Input: part model. Units: mm. Frame: model coordinates. A direction names the side the tool comes from. Coordinates: 2 decimals unless noted, no trailing zeros. Order: outer loops, then holes, each group sorted by start corner. A loop starts at its lowest first (then second) coordinate and runs counter-clockwise, first axis right, second up.
from build123d import *

# Parameters (mm, degrees)
F1_DEPTH = 63.5
F2_DEPTH = 7.62
F4_DEPTH = 7.62
F5_R     = 7.735602
F6_DEPTH = 73.152
F5_R_2   = 7.041534
F7_DEPTH = 76.2


with BuildPart() as f1:
    # F0 (on Front) → F1 (new body)
    with BuildSketch(Plane.XZ):
        with BuildLine():
            Line((-11.978863, 32.654684), (-30.244743, 32.654684))
            Line((-30.244743, 32.654684), (-30.244743, -26.147846))
            Line((-30.244743, -26.147846), (51.452216, -26.147846))
            Line((51.452216, -26.147846), (51.452216, 32.654684))
            Line((51.452216, 32.654684), (33.186335, 32.654684))
            ThreePointArc((33.186335, 32.654684), (10.603736, 10.072085), (-11.978863, 32.654684))
        make_face()
        with BuildLine():
            Line((-4.722234, 32.654684), (-11.978863, 32.654684))
            ThreePointArc((-11.978863, 32.654684), (10.603736, 10.072085), (33.186335, 32.654684))
            Line((33.186335, 32.654684), (25.929707, 32.654684))
            ThreePointArc((25.929707, 32.654684), (10.603736, 17.328714), (-4.722234, 32.654684))
        make_face()
    extrude(amount=F1_DEPTH)

    # F0 (on Front) → F2 (join)
    with BuildSketch(Plane.XZ):
        with BuildLine():
            Line((-4.722234, 32.654684), (-11.978863, 32.654684))
            ThreePointArc((-11.978863, 32.654684), (10.603736, 10.072085), (33.186335, 32.654684))
            Line((33.186335, 32.654684), (25.929707, 32.654684))
            ThreePointArc((25.929707, 32.654684), (10.603736, 17.328714), (-4.722234, 32.654684))
        make_face()
    extrude(amount=-F2_DEPTH)

    # F3 (on face) → F4 (join)
    with BuildSketch(Plane.XZ.offset(63.5)):
        with BuildLine():
            ThreePointArc((-11.5002, 32.654684), (10.603736, 10.550748), (32.707673, 32.654684))
            Line((32.707673, 32.654684), (25.929707, 32.654684))
            ThreePointArc((25.929707, 32.654684), (10.603736, 17.328714), (-4.722234, 32.654684))
            Line((-4.722234, 32.654684), (-11.5002, 32.654684))
        make_face()
    extrude(amount=F4_DEPTH)

    # F5 (on face) → F6 (cut)
    with BuildSketch(Plane.XY.offset(32.654684)):
        with Locations((39.744381, -30.362099)):
            Circle(F5_R)
    extrude(amount=-F6_DEPTH, mode=Mode.SUBTRACT)

    # F5 (on face) → F7 (cut)
    with BuildSketch(Plane.XY.offset(32.654684)):
        with Locations((-19.937346, -31.404577)):
            Circle(F5_R_2)
        with Locations((39.744381, -30.362099)):
            Circle(F5_R)
    extrude(amount=-F7_DEPTH, mode=Mode.SUBTRACT)


solid = f1.part
Item 1: Pin query (flat end, axial travel): pin 1 Ø17.5 at (x, z) = (27.5, -0.5) entering from -Y; pin 2 Ø5 at (x, z) = (-19.5, -17) entering from +Y; pin 3 Ø11.5 at (x, y) = (-19.94, -31.4) entering from +Z. Return the tip coordinate at first contact, or that it passes through.
Response values:
pin 1: stops at y = -63.5
pin 2: stops at y = 0
pin 3: passes through
Item 2: Ray query, probe 1 along X at (y, z) = (-28.5, -12.5); probe 2 along Y at (x, z) = (8, -7.5); probe 3 along X at (y, z) = (-36, -0.5). Return the intervals inside material, ascending.
Response values:
probe 1: x = -30.24 to -26.35, -13.52 to 32.24, 47.25 to 51.45
probe 2: y = -63.5 to 0
probe 3: x = -30.24 to -25.27, -14.6 to 34.45, 45.04 to 51.45
Item 3: Cut plane A-A on z = 25.5. Return loops of the section in (x, y), then the cut area to 3 significant figures.
Response values:
outline: (-30.24, -63.5) - (-10.31, -63.5) - (-10.31, -71.12) - (-2.95, -71.12) - (-2.95, 7.62) - (-10.82, 7.62) - (-10.82, 0) - (-30.24, 0) - close; (24.16, -71.12) - (31.52, -71.12) - (31.52, -63.5) - (51.45, -63.5) - (51.45, 0) - (32.02, 0) - (32.02, 7.62) - (24.16, 7.62) - close; hole circle Ø14.08 at (-19.94, -31.4); hole circle Ø15.47 at (39.74, -30.36)
area: 3,350 mm2
Item 4: Access query for faces 1 (the face through (10.118, -67.257, 10.556)), 2 (the face through (30, -31, 32.655)), 3 (the face through (10.107, 3.757, 10.078)). Directions: +Z, -Z, +X, -X, +Y, -Y. A direction counts if a zero-diameter tool reaches every point of the face in a straight line with its end or side. Return the directions, or none.
Response values:
face 1: -Z, -Y
face 2: +Z, +X, -X, +Y, -Y
face 3: -Z, +Y
Item 5: Cut plane B-B on y = -28.5. Return loops of the section in (x, z), then the cut area to 3 significant figures.
Response values:
outline: (-30.24, -26.15) - (-26.35, -26.15) - (-26.35, 32.65) - (-30.24, 32.65) - close; (-13.52, -26.15) - (32.24, -26.15) - (32.24, 32.65) - (25.93, 32.65) arc R15.33 cw to (-4.72, 32.65) - (-13.52, 32.65) - close; (47.25, -26.15) - (51.45, -26.15) - (51.45, 32.65) - (47.25, 32.65) - close
area: 2,800 mm2
Item 6: Cut plane C-C on z = 13. Return loops of the section in (x, y).
Response values:
outline: (-30.24, -63.5) - (0.49, -63.5) - (0.49, -71.12) - (20.72, -71.12) - (20.72, -63.5) - (51.45, -63.5) - (51.45, 0) - (21.72, 0) - (21.72, 7.62) - (-0.52, 7.62) - (-0.52, 0) - (-30.24, 0) - close; hole circle Ø14.08 at (-19.94, -31.4); hole circle Ø15.47 at (39.74, -30.36)
Item 7: Cut plane D-D on x = 22.5. Return loops of the section in (y, z).
Response values:
outline: (-71.12, 14.03) - (-63.5, 14.03) - (-63.5, -26.15) - (0, -26.15) - (0, 13.46) - (7.62, 13.46) - (7.62, 22.99) - (-71.12, 22.99) - close
